from build123d import *

# Parameters (mm, degrees)
BOSS_EXTRUDE1_DEPTH     = 95
BOSS_EXTRUDE2_START     = -30
SKETCH2_3_R             = 12.5
BOSS_EXTRUDE2_DEPTH     = 63.333333333
EXTRUDE_THIN1_DEPTH     = 115
SKETCH5_W               = 50
SKETCH5_H               = 20
BOSS_EXTRUDE3_DEPTH     = 230
CUT_EXTRUDE2_DEPTH      = 320.256949807
CUT_EXTRUDE2_DEPTH_BACK = 320.256949807
SKETCH5_3_R             = 5
CUT_EXTRUDE1_START      = -30
CUT_EXTRUDE1_OUTLINE_R  = 8.5
CUT_EXTRUDE1_DEPTH      = 125
RIB1_START              = -2.5
RIB1_DEPTH              = 5
FILLET1_R               = 10


# Read off the part's stored shape, not the designer's step: Cut-Extrude1, Rib1
with BuildPart() as part:
    # Sketch2 → Boss-Extrude1 (new body)
    with BuildSketch(Plane(origin=(0, 0, 0), x_dir=(1, 0, 0), z_dir=(0, 1, 0))):
        with BuildLine():
            Line((43.336618465, 6), (48.75, 6))
            Line((48.75, 6), (48.75, -6))
            Line((48.75, -6), (43.336618465, -6))
            ThreePointArc((43.336618465, -6), (-43.75, 0), (43.336618465, 6))
        make_face()
    extrude(amount=BOSS_EXTRUDE1_DEPTH)



with BuildPart() as body_2:
    # Sketch2<3> → Boss-Extrude2 (new body)
    with BuildSketch(Plane(origin=(0, 0, 0), x_dir=(1, 0, 0), z_dir=(0, 1, 0)).offset(BOSS_EXTRUDE2_START)):
        with Locations(Location((175, 0, 0), (0, 0, 270))):
            Circle(SKETCH2_3_R)
    extrude(amount=BOSS_EXTRUDE2_DEPTH)


with BuildPart() as part_1:
    add(part.part)

    add(body_2.part)  # Extrude-Thin1 merges body 2
    # Sketch3 → Extrude-Thin1 (add, symmetric)
    with BuildSketch(Plane.XY):
        Polygon((-43.75, 0), (99.247392222, 0), (135, -30), (187.5, -30), (187.5, -24), (137.183821406, -24), (101.431213628, 6), (-43.75, 6), align=None)
    extrude(amount=EXTRUDE_THIN1_DEPTH, both=True)

    # Sketch5 → Boss-Extrude3 (add)
    with BuildSketch(Plane.XY.offset(115)):
        with Locations((175, -20)):
            Rectangle(SKETCH5_W, SKETCH5_H)
    extrude(amount=-BOSS_EXTRUDE3_DEPTH)

    # Sketch5<3> → Cut-Extrude2 (cut, two sides: drawn at the far end of the back side and taken through both)
    with BuildSketch(Plane.XY.offset(115).offset(-CUT_EXTRUDE2_DEPTH_BACK)):
        with Locations((160, -20)):
            Circle(SKETCH5_3_R)
    extrude(amount=CUT_EXTRUDE2_DEPTH + CUT_EXTRUDE2_DEPTH_BACK, mode=Mode.SUBTRACT)

    # Cut-Extrude1 outline → Cut-Extrude1 (cut)
    with BuildSketch(Plane(origin=(0, 0, 0), x_dir=(1, 0, 0), z_dir=(0, 1, 0)).offset(CUT_EXTRUDE1_START)):
        with BuildLine():
            ThreePointArc((177.232142857, 12.299086887), (184.59561842, 8.010874306), (187.5, 0))
            ThreePointArc((187.5, 0), (184.59561842, -8.010874306), (177.232142857, -12.299086887))
            Line((177.232142857, -12.299086887), (150, -17.241407705))
            Line((150, -17.241407705), (150, -115))
            Line((150, -115), (200, -115))
            Line((200, -115), (200, 115))
            Line((200, 115), (150, 115))
            Line((150, 115), (150, 17.241407705))
            Line((150, 17.241407705), (177.232142857, 12.299086887))
        make_face()
        with BuildLine():
            Line((7.8125, 43.046804106), (150, 17.241407705))
            Line((150, 17.241407705), (150, 115))
            Line((150, 115), (-43.75, 115))
            Line((-43.75, 115), (-43.75, -4.5e-08))
            ThreePointArc((-43.75, -4.5e-08), (-28.038060087, 33.584664455), (7.8125, 43.046804106))
        make_face()
        with BuildLine():
            Line((150, -115), (150, -17.241407705))
            Line((150, -17.241407705), (7.8125, -43.046804106))
            ThreePointArc((7.8125, -43.046804106), (-28.038060053, -33.584664483), (-43.75, -4.5e-08))
            Line((-43.75, -4.5e-08), (-43.75, -115))
            Line((-43.75, -115), (150, -115))
        make_face()
        with Locations((175, 0)):
            Circle(CUT_EXTRUDE1_OUTLINE_R)
        with BuildLine():
            Line((45.75, 3), (39.636630785, 3))
            ThreePointArc((39.636630785, 3), (-39.75, 0), (39.636630785, -3))
            Line((39.636630785, -3), (45.75, -3))
            Line((45.75, -3), (45.75, 3))
        make_face()
    extrude(amount=CUT_EXTRUDE1_DEPTH, mode=Mode.SUBTRACT)

    # Rib1 outline → Rib1 (add)
    with BuildSketch(Plane.XY.offset(RIB1_START)):
        Polygon((158.05144817, 33.333333333), (84.559976627, 95), (48.75, 95), (48.75, 6), (101.431213628, 6), (137.183821406, -24), (150, -24), (150, -10), (164, -10), (164, 33.333333333), align=None)
    extrude(amount=RIB1_DEPTH)

    # Fillet1
    fillet1_edges = [part_1.edges().sort_by_distance(p)[0] for p in [
        (150, -10, 9.870703853),
        (137.183821406, -24, -11.033698381),
        (101.431213628, 6, -14.278041998),
        (158.05144817, 33.333333333, 0),
        (84.559976627, 95, 0),
        (150, -10, -9.870703853),
        (99.247392222, 0, 0),
        (101.431213628, 6, 14.278041998),
        (137.183821406, -24, 11.033698381),
        (135, -30, 0),
    ]]
    fillet(fillet1_edges, radius=FILLET1_R)


solid = part_1.part
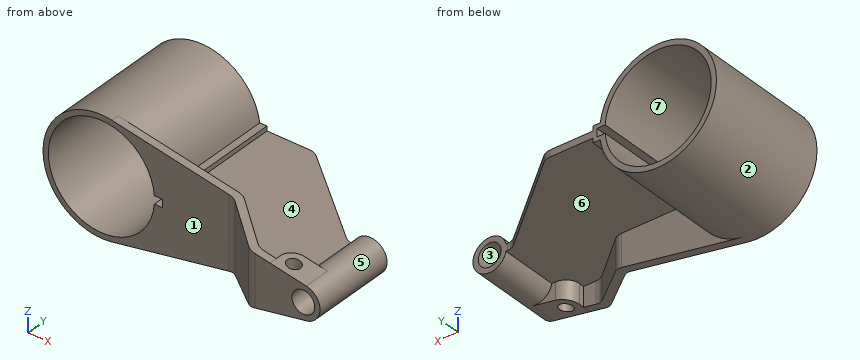
Could you check a few things on this model? Use its own coordinates, in mm. Face numbers are marked on the shaded views. A direction names the side the tool comes from. Round coordinates to 2 decimals unless told otherwise and drop trailing zeros. Order: outer loops, then holes, each group sorted by start corner. A loop starts at its lowest first (then second) coordinate and runs counter-clockwise, first axis right, second up.
(1) Imagine slicing it at C-C (z = -33). Write out the boundary of the cut face in (x, y).
Response values:
outline: (-28.72, 0) - (-22.16, 0) - (-22.16, 95) - (-28.72, 95) - close; (22.16, 0) - (63.17, 0) - (63.17, 6) - (28.72, 6) - (28.72, 95) - (22.16, 95) - close
(2) Imagine slicing it at A-A (x = 0). Write out the boundary of the cut face in (y, z), plus the area to 3 significant figures.
Response values:
outline: (0, -43.75) - (95, -43.75) - (95, -39.75) - (0, -39.75) - close; (0, 39.75) - (95, 39.75) - (95, 43.75) - (0, 43.75) - close
area: 760 mm2
(3) Which directions (+Z, -Z, +X, -X, +Y, -Y) give clear straight access to the entire face, cutting with the end or side of a thin tool? Please do the marked faces 4, 5, 6 and 7.
Response values:
face 4: +Z, +Y
face 5: +Y
face 6: -Z, +Y
face 7: +Y, -Y
(4) I'm going to push flat-ended pins straight in: pin 1 (10.5 mm diameter, centred on x = 170, z = 11, fed in from +Y); pin 2 (3 mm diameter, centred on y = 60, z = 31, fed in from -X); pin 3 (6 mm diameter, centred on y = 58.5, z = -7.5, fed in from +X); pin 4 (8 mm diameter, centred on x = -2.5, y = 41.5, fed in from +Z). Where does each tip first touch, or does it pass through?
Response values:
pin 1: stops at y = 33.33
pin 2: stops at x = -32.31
pin 3: stops at x = 48.75
pin 4: stops at z = 43.75
(5) If we mould it in two halves opening along Z, with no side actions, what happens to the marked faces 1, 2 and 3? For each: released by +Z, released by -Z, zero draft, split by the parting line, or undercut.
Response values:
face 1: zero draft
face 2: split by the parting line
face 3: undercut
(6) Imagine slicing it at D-D (y = 55). Write out the boundary of the cut face in (x, z).
Response values:
outline: (43.34, -6) - (48.75, -6) - (48.75, -2.5) - (132.23, -2.5) - (132.23, 2.5) - (48.75, 2.5) - (48.75, 6) - (43.34, 6) arc R43.75 ccw (long way) to start; hole (39.64, -3) - (45.75, -3) - (45.75, 3) - (39.64, 3) arc R39.75 ccw (long way) to start
(7) Imagine slicing it at B-B (y = 22). Write out the boundary of the cut face in (x, z).
Response values:
outline: (43.34, -6) - (48.75, -6) - (48.75, -2.5) - (162.75, -2.5) arc R12.5 ccw (long way) to (162.75, 2.5) - (48.75, 2.5) - (48.75, 6) - (43.34, 6) arc R43.75 ccw (long way) to start; hole (39.64, -3) - (45.75, -3) - (45.75, 3) - (39.64, 3) arc R39.75 ccw (long way) to start; hole circle Ø17 at (175, 0)
(8) Please list where these lines run through material, in increasing order: line 1 along Z through (x, y) = (0, 30); line 2 along X through (y, z) = (-20, -9); line 3 along Y through (x, z) = (143, 7.5).
Response values:
line 1: z = -43.75 to -39.75, 39.75 to 43.75
line 2: x = 123.08 to 132.42, 150 to 155, 165 to 183.67
line 3: y = -30 to -24
